from build123d import *

# Parameters (mm, degrees)
SKETCH2_R           = 2.5
BOSS_EXTRUDE1_DEPTH = 0.5
BOSS_EXTRUDE2_DEPTH = 8
FILLET1_R           = 0.5


with BuildPart() as part:
    # Sketch2 → Boss-Extrude1 (new body)
    with BuildSketch(Plane(origin=(0, 0, 0), x_dir=(1, 0, 0), z_dir=(0, 1, 0))):
        with Locations(Location((0, 0, 0), (0, 0, 270))):
            Circle(SKETCH2_R)
    extrude(amount=BOSS_EXTRUDE1_DEPTH)

    # Sketch3 → Boss-Extrude2 (add)
    with BuildSketch(Plane(origin=(0, 0.5, 0), x_dir=(1, 0, 0), z_dir=(0, 1, 0))):
        with BuildLine():
            Line((1.5, 2), (-1.5, 2))
            ThreePointArc((-1.5, 2), (-2.236067977, 1.118033989), (-2.5, 0))
            Line((-2.5, 0), (-0.75, 0))
            ThreePointArc((-0.75, 0), (0, 0.75), (0.75, 0))
            Line((0.75, 0), (2.5, 0))
            ThreePointArc((2.5, 0), (2.236067977, 1.118033989), (1.5, 2))
        make_face()
        with BuildLine():
            Line((-0.75, 0), (-2.5, 0))
            ThreePointArc((-2.5, 0), (-2.236067977, -1.118033989), (-1.5, -2))
            Line((-1.5, -2), (1.5, -2))
            ThreePointArc((1.5, -2), (2.236067977, -1.118033989), (2.5, 0))
            Line((2.5, 0), (0.75, 0))
            ThreePointArc((0.75, 0), (0, -0.75), (-0.75, 0))
        make_face()
    extrude(amount=BOSS_EXTRUDE2_DEPTH)

    # Fillet1
    # the kernel refuses this fillet: 0.5 mm, written as the material it takes off along each edge
    with BuildSketch(Plane(origin=(-1.5, 0.5, -2), x_dir=(-0.7756085685899518, 0, 0.6312141857799506), z_dir=(0, 1, 0)), Plane(origin=(1.5, 0.5, 2), x_dir=(0.7756085685899534, 0, -0.6312141857799487), z_dir=(0, 1, 0))) as fillet1_piece_1:
        with BuildLine():
            CenterArc((0.178227934, 0.499607683), FILLET1_R, 230.860240122, 41.409622109)
            Line((-0.137379159, 0.111803399), (0, 0))
            ThreePointArc((0, 0), (0.099015519, -0.001961584), (0.198031037, 0))
        make_face()
    extrude(amount=8.495077593, mode=Mode.SUBTRACT)
    with BuildSketch(Plane(origin=(1.5, 0.5, -2), x_dir=(0.7756085685899526, 0, 0.6312141857799497), z_dir=(0, 1, 0)), Plane(origin=(-1.5, 0.5, 2), x_dir=(-0.7756085685899534, 0, -0.6312141857799487), z_dir=(0, 1, 0))) as fillet1_piece_2:
        with BuildLine():
            CenterArc((0.178227934, -0.499607683), FILLET1_R, 87.730137768, 41.409622109)
            Line((-0.137379159, -0.111803399), (0, 0))
            ThreePointArc((0, 0), (0.099015519, 0.001961584), (0.198031037, 0))
        make_face()
    extrude(amount=8.495077593, mode=Mode.SUBTRACT)


solid = part.part
Read the model definition and answer for the solid it produces. Units are mm, in the model's axes. A direction names the side the tool comes from. Coordinates: 2 decimals unless noted, no trailing zeros. Loops run counter-clockwise (first coordinate to the right, second up) from the corner with the lowest first, then second, coordinate; pieces in that order, holes last. Notation, with made-up numbers: (82.25, 36) - (121.25, 36) arc R22 cw to (121.25, 71) - close; hole circle Ø4 at (38, 47.5). An arc over 180 degrees is marked (long way). Answer in a Markdown table with one row per item.
Q1. For faces 1 (the flat face through (0, 4, 2)), 2 (the cylindrical face through (-0.75, 4.44, 0.03)), 3 (the flat face through (0, 4, -2)), determine the directions among +Z, -Z, +X, -X, +Y, -Y from which every point of the face is accessible in a straight line to the end or side of a thin tool.
Here are the results:
| item | result |
|---|---|
| face 1 | +Z, +X, -X, +Y |
| face 2 | +Y |
| face 3 | -Z, +X, -X, +Y |
Q2. Given P1, Ø1.5, axis at x = 1.5, y = 4, coming from the -Z side; P2, Ø1, axis at x = -1.5, y = 7.5, coming from the +Z side, each flat-ended and moving along its own axis, determine where each tip first touches the part or whether it passes through.
Here are the results:
| item | result |
|---|---|
| P1 | stops at z = -2 |
| P2 | stops at z = 2 |
Q3. Straight lines are drawn through the part: line 1 along Z through (x, y) = (0, 2.75); line 2 along Z through (x, y) = (1.65, 2.25); line 3 along Z through (x, y) = (-1.3, 5.5). For each, find the intervals that lie inside material, in ascending order. Write a range as [from, to].
Here are the results:
| item | result |
|---|---|
| line 1 | z = [-2, -0.75], [0.75, 2] |
| line 2 | z = [-1.88, 1.88] |
| line 3 | z = [-2, 2] |
Q4. Find section C-C on x = 0. Write down the section's boundary in (y, z), plus the area to 3 significant figures.
Here are the results:
| item | result |
|---|---|
| outline | (0, -2.5) - (0.5, -2.5) - (0.5, -2) - (8.5, -2) - (8.5, -0.75) - (0.5, -0.75) - (0.5, 0.75) - (8.5, 0.75) - (8.5, 2) - (0.5, 2) - (0.5, 2.5) - (0, 2.5) - close |
| area | 22.5 mm^2 |
Q5. Find section A-A on y = 6.75. Write down the section's boundary in (x, z) (3 decimals), plus the area to 3 significant figures.
Here are the results:
| item | result |
|---|---|
| outline | (-1.654, -1.875) arc R0.5 ccw to (-1.323, -2) - (1.323, -2) arc R0.5 ccw to (1.654, -1.875) arc R2.5 ccw to (1.654, 1.875) arc R0.5 ccw to (1.323, 2) - (-1.323, 2) arc R0.5 ccw to (-1.654, 1.875) arc R2.5 ccw to start; hole circle Ø1.5 at (0, 0) |
| area | 15.8 mm^2 |
Q6. Find section B-B on z = 0. Write down the section's boundary in (x, y), plus the area to 3 significant figures.
Here are the results:
| item | result |
|---|---|
| outline | (-2.5, 0) - (2.5, 0) - (2.5, 8.5) - (0.75, 8.5) - (0.75, 0.5) - (-0.75, 0.5) - (-0.75, 8.5) - (-2.5, 8.5) - close |
| area | 30.5 mm^2 |
Q7. Find section D-D on x = 1.1. Write down the section's boundary in (y, z) (3 decimals), plus the area to 3 significant figures.
Here are the results:
| item | result |
|---|---|
| outline | (0, -2.245) - (0.5, -2.245) - (0.5, -2) - (8.5, -2) - (8.5, 2) - (0.5, 2) - (0.5, 2.245) - (0, 2.245) - close |
| area | 34.2 mm^2 |
